```python
from build123d import *

# Parameters (mm, degrees)
EXTRUDE_3_DEPTH = 10
EXTRUDE_4_DEPTH = 20


with BuildPart() as part:
    # 草圖1 → 填料-伸長3 (new body)
    with BuildSketch(Plane(origin=(0, 0, 0), x_dir=(1, 0, 0), z_dir=(0, 1, 0))):
        with BuildLine():
            Line((-60, 50), (60, 50))
            ThreePointArc((60, 50), (110, 0), (60, -50))
            Line((60, -50), (-60, -50))
            ThreePointArc((-60, -50), (-110, 0), (-60, 50))
        make_face()
        with BuildLine():
            Line((-60, -30), (60, -30))
            ThreePointArc((60, -30), (90, 0), (60, 30))
            Line((60, 30), (-60, 30))
            ThreePointArc((-60, 30), (-90, 0), (-60, -30))
        make_face(mode=Mode.SUBTRACT)
    extrude(amount=EXTRUDE_3_DEPTH)

    # 草圖4 → 填料-伸長4 (add)
    # profile 1 of 2: a face of its own
    with BuildSketch(Plane(origin=(0, 0, 0), x_dir=(1, 0, 0), z_dir=(0, 1, 0))):
        with BuildLine():
            Line((-60, 50), (60, 50))
            ThreePointArc((60, 50), (110, 0), (60, -50))
            Line((60, -50), (-60, -50))
            ThreePointArc((-60, -50), (-110, 0), (-60, 50))
        make_face()
        with BuildLine():
            ThreePointArc((60, -47), (107, 0), (60, 47))
            Line((60, 47), (-60, 47))
            ThreePointArc((-60, 47), (-107, 0), (-60, -47))
            Line((-60, -47), (60, -47))
        make_face(mode=Mode.SUBTRACT)
    # profile 2 of 2: a face of its own
    with BuildSketch(Plane(origin=(0, 0, 0), x_dir=(1, 0, 0), z_dir=(0, 1, 0))):
        with BuildLine():
            Line((-60, 33), (60, 33))
            ThreePointArc((60, 33), (93, 0), (60, -33))
            Line((60, -33), (-60, -33))
            ThreePointArc((-60, -33), (-93, 0), (-60, 33))
        make_face()
        with BuildLine():
            ThreePointArc((-60, 30), (-90, 0), (-60, -30))
            Line((-60, -30), (60, -30))
            ThreePointArc((60, -30), (90, 0), (60, 30))
            Line((60, 30), (-60, 30))
        make_face(mode=Mode.SUBTRACT)
    extrude(amount=EXTRUDE_4_DEPTH)


solid = part.part
```
Input: part model. Units: mm. Frame: model coordinates. A direction names the side the tool comes from. Round coordinates to 2 decimals unless told otherwise and drop trailing zeros. Loops run counter-clockwise (first coordinate to the right, second up) from the corner with the lowest first, then second, coordinate; pieces in that order, holes last. Notation, with made-up numbers: (82, -4.75) -> (124, -4.75) arc R21 cw to (124, 13.25) -> close; hole circle Ø8 at (86.25, 13.25). An arc over 180 degrees is marked (long way). One line per item, written item: value.
(1) Section D-D (z = -36.5). Return the cut outline in (x, y).
Geometry check:
outline: (-94.17, 0) -> (94.17, 0) -> (94.17, 20) -> (89.61, 20) -> (89.61, 10) -> (-89.61, 10) -> (-89.61, 20) -> (-94.17, 20) -> close
(2) Set-up query: faces 1 (the face through (-89.993, 9.86, -0.66)), 2 (the face through (1, 20, 48)), 3 (the face through (92.99, 14.93, -0.73)). Return all of +Z, -Z, +X, -X, +Y, -Y with unobstructed straight access to the full face (end or side cutting, diameter ignored); none if empty.
Geometry check:
face 1: +Y, -Y
face 2: +Z, -Z, +X, -X, +Y
face 3: +Y
(3) Section B-B (z = 0). Return the cut outline in (x, y).
Geometry check:
outline: (-110, 0) -> (-90, 0) -> (-90, 20) -> (-93, 20) -> (-93, 10) -> (-107, 10) -> (-107, 20) -> (-110, 20) -> close; (90, 0) -> (110, 0) -> (110, 20) -> (107, 20) -> (107, 10) -> (93, 10) -> (93, 20) -> (90, 20) -> close
(4) Pin query (flat end, axial travel): pin 1 (4 mm diameter, centred on x = -69, y = 4, fed in from -Z); pin 2 (4 mm diameter, centred on y = 2, z = -6, fed in from +X); pin 3 (5 mm diameter, centred on x = 68, y = 17, fed in from -Z); pin 4 (12 mm diameter, centred on x = -70, z = 26, fed in from -Y). Return the tip coordinate at first contact, or that it passes through.
Geometry check:
pin 1: z = -49.51
pin 2: x = 109.84
pin 3: z = -49.7
pin 4: y = 0
(5) Section C-C (x = 13.5). Return the cut outline in (y, z), plus the area to 3 significant figures.
Geometry check:
outline: (0, -50) -> (20, -50) -> (20, -47) -> (10, -47) -> (10, -33) -> (20, -33) -> (20, -30) -> (0, -30) -> close; (0, 30) -> (20, 30) -> (20, 33) -> (10, 33) -> (10, 47) -> (20, 47) -> (20, 50) -> (0, 50) -> close
area: 520 mm2
(6) Mould query, pull axis X, two halves, no side actions, for faces 4 (the face through (-109.988, 9.86, 1.099)), 5 (the face through (109.988, 9.86, -1.099)), 6 (the face through (89.993, 9.86, 0.66)), 7 (the face through (1, 10, 50)). Classes: pulls with the +X half, pulls with the -X half, needs draft (parallel to the pull), parting line crosses it, or undercut.
Geometry check:
face 4: pulls with the -X half
face 5: pulls with the +X half
face 6: undercut
face 7: needs draft
(7) Material intervals for line 1 (Z direction, x = 46, y = 18.5); line 2 (Z direction, x = -26, y = 9.25); line 3 (X direction, y = 14, z = -15), sorted ascending. Write a range as [from, to].
Geometry check:
line 1: [-50, -47], [-33, -30], [30, 33], [47, 50]
line 2: [-50, -30], [30, 50]
line 3: [-107.7, -104.54], [-89.39, -85.98], [85.98, 89.39], [104.54, 107.7]
(8) Section A-A (y = 16). Return the cut outline in (x, z), plus the area to 3 significant figures.
Geometry check:
outline: (-60, -50) -> (60, -50) arc R50 ccw to (60, 50) -> (-60, 50) arc R50 ccw to start; (-60, -33) -> (60, -33) arc R33 ccw to (60, 33) -> (-60, 33) arc R33 ccw to start; hole (-60, -47) -> (60, -47) arc R47 ccw to (60, 47) -> (-60, 47) arc R47 ccw to start; hole (-60, -30) -> (60, -30) arc R30 ccw to (60, 30) -> (-60, 30) arc R30 ccw to start
area: 2,950 mm2
